Work out the finished part from the listing and answer in its coordinate system (mm). Coordinates: 2 decimals unless noted, no trailing zeros. Order: outer loops, then holes, each group sorted by start corner. A loop starts at its lowest first (then second) coordinate and runs counter-clockwise, first axis right, second up. Notation, with made-up numbers: (-1.5, 78) - (19.5, 78) arc R9 cw to (19.5, 95) - close; hole circle Ø2 at (-18.5, 22). An arc over 180 degrees is marked (long way). Answer as a JSON object with one key per item and string values. Group by question number.
1) Section B-B (y = 13) is taken. Give the vertices of the cut face in (x, z), plus the area to 3 significant figures.
2) Section A-A (z = 1.2) is taken. Count the separate pieces of the cut face and the enclosed holes in it, plus the area to 3 significant figures.
3) This flat-tipped pin is pushed along its axis until it touches: P1, Ø0.6, axis at x = 1, z = 1.5, coming from the -Y side. Where does it stop, or does it pass through?
4) Find the intervals of material crossed by line 1 along Y through (x, z) = (11.5, 1.25); line 2 along X through (y, z) = (75, 0.5); line 3 along X through (y, z) = (-17, 0.9), in increasing order.
from build123d import *

# Parameters (mm, degrees)
CROQUIS1_R              = 1.5
SALIENTE_EXTRUIR1_DEPTH = 2
CROQUIS2_W              = 25
CROQUIS2_H              = 3
CROQUIS2_W_2            = 21.071847778
CORTAR_EXTRUIR1_DEPTH   = 2
REDONDEO2_R             = 1
REDONDEO1_R             = 3


with BuildPart() as part:
    # Croquis1 → Saliente-Extruir1 (new body)
    with BuildSketch(Plane.XY):
        Polygon((-17.535923889, 31.688251973), (-15, 80), (0, 83), (15, 80), (17.535923889, 31.688251973), (17.535923889, -31.688251973), (15, -80), (0, -83), (-15, -80), (-17.535923889, -31.688251973), align=None)
        with Locations((-11.5, 75)):
            Circle(CROQUIS1_R, mode=Mode.SUBTRACT)
        with Locations((11.5, 75)):
            Circle(CROQUIS1_R, mode=Mode.SUBTRACT)
        with Locations((14, 30)):
            Circle(CROQUIS1_R, mode=Mode.SUBTRACT)
        with Locations((-14, 30)):
            Circle(CROQUIS1_R, mode=Mode.SUBTRACT)
        with Locations((-14, -30)):
            Circle(CROQUIS1_R, mode=Mode.SUBTRACT)
        with Locations((14, -30)):
            Circle(CROQUIS1_R, mode=Mode.SUBTRACT)
        with Locations((-11.5, -75)):
            Circle(CROQUIS1_R, mode=Mode.SUBTRACT)
        with Locations((11.5, -75)):
            Circle(CROQUIS1_R, mode=Mode.SUBTRACT)
    extrude(amount=SALIENTE_EXTRUIR1_DEPTH)

    # Croquis2 → Cortar-Extruir1 (cut)
    with BuildSketch(Plane.XY.offset(2)):
        Polygon((-10.097096622, 80.980580676), (-6, 67.5), (6, 67.5), (10.097096622, 80.980580676), (0, 83), align=None)
        Polygon((-10, 64.432841453), (-11.051306944, 40.455878474), (-2, 52.07053953), align=None)
        Polygon((2, 52.07053953), (10, 64.432841453), (11.051306944, 40.455878474), align=None)
        Polygon((0, 30), (-8, 37.5), (0, 47.7656212), (8, 37.5), align=None)
        Polygon((-10.535923889, 18), (10.535923889, 18), (0, 4.5), align=None)
        with Locations((0, 23.5)):
            Rectangle(CROQUIS2_W, CROQUIS2_H)
        Rectangle(CROQUIS2_W_2, CROQUIS2_H)
        Polygon((0, -4.5), (10.535923889, -18), (-10.535923889, -18), align=None)
        with Locations((0, -23.5)):
            Rectangle(CROQUIS2_W, CROQUIS2_H)
        Polygon((8, -37.5), (0, -47.7656212), (-8, -37.5), (0, -30), align=None)
        Polygon((11.051306944, -40.455878474), (2, -52.07053953), (10, -64.432841453), align=None)
        Polygon((-2, -52.07053953), (-10, -64.432841453), (-11.051306944, -40.455878474), align=None)
        Polygon((10.097096622, -80.980580676), (0, -83), (-10.097096622, -80.980580676), (-6, -67.5), (6, -67.5), align=None)
    extrude(amount=-CORTAR_EXTRUIR1_DEPTH, mode=Mode.SUBTRACT)

    # Redondeo2
    redondeo2_edges = [part.edges().sort_by_distance(p)[0] for p in [
        (-12.5, 22, 1),
        (-12.5, 25, 1),
        (12.5, 25, 1),
        (12.5, 22, 1),
        (11.051306944, 40.455878474, 1),
        (2, 52.07053953, 1),
        (10, 64.432841453, 1),
        (-10, 64.432841453, 1),
        (-2, 52.07053953, 1),
        (-11.051306944, 40.455878474, 1),
        (0, 47.7656212, 1),
        (8, 37.5, 1),
        (0, 30, 1),
        (-8, 37.5, 1),
        (-10.535923889, -18, 1),
        (0, -4.5, 1),
        (10.535923889, -18, 1),
        (-10.535923889, 1.5, 1),
        (10.535923889, 1.5, 1),
        (10.535923889, -1.5, 1),
        (-10.535923889, -1.5, 1),
        (12.5, -25, 1),
        (-12.5, -25, 1),
        (-12.5, -22, 1),
        (12.5, -22, 1),
        (0, 4.5, 1),
        (-10.535923889, 18, 1),
        (10.535923889, 18, 1),
        (11.051306944, -40.455878474, 1),
        (10, -64.432841453, 1),
        (2, -52.07053953, 1),
        (-8, -37.5, 1),
        (0, -30, 1),
        (8, -37.5, 1),
        (0, -47.7656212, 1),
        (-11.051306944, -40.455878474, 1),
        (-2, -52.07053953, 1),
        (-10, -64.432841453, 1),
    ]]
    fillet(redondeo2_edges, radius=REDONDEO2_R)

    # Redondeo1
    # the kernel refuses this fillet: 3 mm, written as the material it adds along each edge
    with BuildSketch(Plane(origin=(-6, -67.5, 2), x_dir=(-0.29079205959554133, -0.956786276070149, 0), z_dir=(0, 0, -1)), Plane(origin=(6, -67.5, 2), x_dir=(-1, 0, 0), z_dir=(0, 0, -1)), Plane(origin=(6, 67.5, 2), x_dir=(0.2907920595955413, 0.9567862760701489, 0), z_dir=(0, 0, -1)), Plane(origin=(-6, 67.5, 2), x_dir=(1, 0, 0), z_dir=(0, 0, -1))) as redondeo1_piece_1:
        with BuildLine():
            CenterArc((REDONDEO1_R * 0.741239666728, -REDONDEO1_R), REDONDEO1_R, 90, 73.09461858)
            Line((-REDONDEO1_R * 0.215546609342, -REDONDEO1_R * 0.709207940404), (0, 0))
            Line((0, 0), (REDONDEO1_R * 0.741239666728, 0))
        make_face()
    extrude(amount=2)
    # the kernel refuses this fillet: 3 mm, written as the material it takes off along each edge
    with BuildSketch(Plane(origin=(15, -80, -5.826545773), x_dir=(-0.9805806756909198, -0.1961161351381855, 0), z_dir=(0, 0, 1)), Plane(origin=(-15, -80, -5.826545773), x_dir=(-0.05241866824073038, 0.9986251965676953, 0), z_dir=(0, 0, 1)), Plane(origin=(15, 80, -5.826545773), x_dir=(0.052418668240731464, -0.9986251965676953, 0), z_dir=(0, 0, 1)), Plane(origin=(-15, 80, -5.826545773), x_dir=(0.9805806756909198, 0.19611613513818563, 0), z_dir=(0, 0, 1))) as redondeo1_2_piece_1:
        with BuildLine():
            CenterArc((REDONDEO1_R * 0.776872769711, -REDONDEO1_R), REDONDEO1_R, 90, 75.685321964)
            Line((-REDONDEO1_R * 0.192079653677, -REDONDEO1_R * 0.752752752875), (0, 0))
            Line((0, 0), (REDONDEO1_R * 0.776872769711, 0))
        make_face()
    extrude(amount=13.653091546, mode=Mode.SUBTRACT)
    with BuildSketch(Plane(origin=(10.097096622, -80.980580676, 8.801127509), x_dir=(-0.29079205959554183, 0.9567862760701488, 0), z_dir=(0, 0, -1)), Plane(origin=(-10.097096622, -80.980580676, 8.801127509), x_dir=(-0.98058067569092, 0.1961161351381849, 0), z_dir=(0, 0, -1)), Plane(origin=(10.097096622, 80.980580676, 8.801127509), x_dir=(0.98058067569092, -0.1961161351381849, 0), z_dir=(0, 0, -1)), Plane(origin=(-10.097096622, 80.980580676, 8.801127509), x_dir=(0.29079205959554244, -0.9567862760701485, 0), z_dir=(0, 0, -1))) as redondeo1_2_piece_2:
        with BuildLine():
            CenterArc((REDONDEO1_R * 0.906817001191, REDONDEO1_R), REDONDEO1_R, 185.595448946, 84.404551054)
            Line((-REDONDEO1_R * 0.0884181467465, REDONDEO1_R * 0.902496152332), (0, 0))
            Line((0, 0), (REDONDEO1_R * 0.906817001191, 0))
        make_face()
    extrude(amount=15.602255018, mode=Mode.SUBTRACT)
    with BuildSketch(Plane(origin=(17.535923889, -31.688251973, -0.196705221), x_dir=(-0.052418668240729306, -0.9986251965676954, 0), z_dir=(0, 0, 1)), Plane(origin=(17.535923889, 31.688251973, -0.196705221), x_dir=(0, -1, 0), z_dir=(0, 0, 1)), Plane(origin=(-17.535923889, -31.688251973, -0.196705221), x_dir=(0, 1, 0), z_dir=(0, 0, 1))) as redondeo1_2_piece_3:
        with BuildLine():
            CenterArc((REDONDEO1_R * 0.0262273628546, -REDONDEO1_R), REDONDEO1_R, 90, 3.004745562)
            Line((-REDONDEO1_R * 0.0261913053861, -REDONDEO1_R * 0.0013748034323), (0, 0))
            Line((0, 0), (REDONDEO1_R * 0.0262273628546, 0))
        make_face()
    extrude(amount=2.393410443, mode=Mode.SUBTRACT)
    with BuildSketch(Plane(origin=(-17.535923889, 31.688251973, -0.196705221), x_dir=(0, -1, 0), z_dir=(0, 0, 1))) as redondeo1_2_piece_4:
        with BuildLine():
            CenterArc((REDONDEO1_R * 0.0262273628546, REDONDEO1_R), REDONDEO1_R, 266.995254438, 3.004745562)
            Line((-REDONDEO1_R * 0.0261913053861, REDONDEO1_R * 0.0013748034323), (0, 0))
            Line((0, 0), (REDONDEO1_R * 0.0262273628546, 0))
        make_face()
    extrude(amount=2.393410443, mode=Mode.SUBTRACT)


solid = part.part
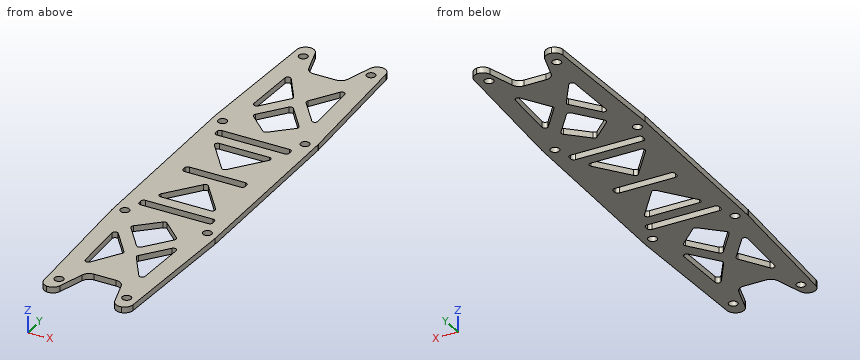
Report:
{
 "1": {"outline": "(-17.54, 0) - (-6.63, 0) - (-6.63, 2) - (-17.54, 2) - close; (6.63, 0) - (17.54, 0) - (17.54, 2) - (6.63, 2) - close", "area": "43.6 mm²"},
 "2": {"separate pieces": "1", "enclosed holes": "19", "area": "3,750 mm²"},
 "3": {"P1": "stops at y = -67.5"},
 "4": {"line 1": "y = -80.43 to -76.5, -73.5 to -25, -22 to 22, 25 to 73.5, 76.5 to 80.43", "line 2": "x = -15.26 to -13, -10 to -8.28, 8.28 to 10, 13 to 15.26", "line 3": "x = -17.54 to -9.49, 9.49 to 17.54"}
}
